from build123d import *

# Parameters (mm, degrees)
SKETCH1_W           = 17.78
SKETCH1_H           = 39.02
BOSS_EXTRUDE1_DEPTH = 2
SKETCH2_R           = 1
CUT_EXTRUDE5_DEPTH  = 10
FILLET4_R           = 7


with BuildPart() as part:
    # Sketch1 → Boss-Extrude1 (new body)
    with BuildSketch(Plane.XY):
        with Locations((8.89, 19.51)):
            Rectangle(SKETCH1_W, SKETCH1_H)
    extrude(amount=BOSS_EXTRUDE1_DEPTH)

    # Sketch2 → Cut-Extrude5 (cut)
    with BuildSketch(Plane.XY.offset(2)):
        with Locations((5.081291963, 2)):
            Circle(SKETCH2_R)
        with Locations((7.621291963, 2)):
            Circle(SKETCH2_R)
        with Locations((10.161291963, 2)):
            Circle(SKETCH2_R)
        with Locations((12.701291963, 2)):
            Circle(SKETCH2_R)
    extrude(amount=-CUT_EXTRUDE5_DEPTH, mode=Mode.SUBTRACT)

    # Fillet4
    fillet4_edges = [part.edges().sort_by_distance(p)[0] for p in [
        (17.78, 0, 1),
        (0, 0, 1),
    ]]
    fillet(fillet4_edges, radius=FILLET4_R)


solid = part.part
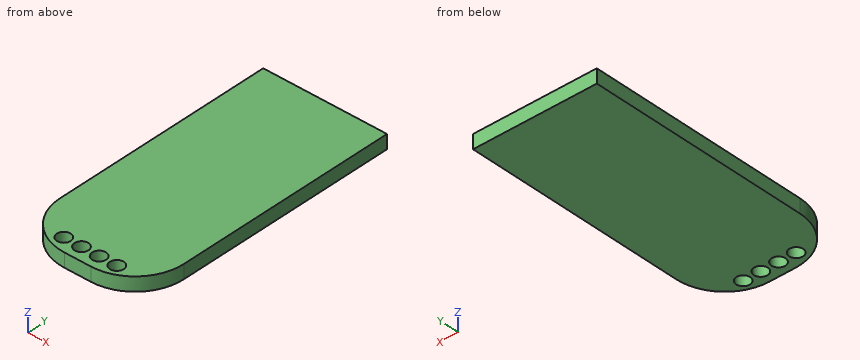
The model under review builds one solid part; all positions refer to its coordinate system, in mm. Round coordinates to 2 decimals unless told otherwise and drop trailing zeros. Loops run counter-clockwise (first coordinate to the right, second up) from the corner with the lowest first, then second, coordinate; pieces in that order, holes last. Notation, with made-up numbers: M -19.5,83 L 2.5,83 A4 ccw 2.5,88 Z; hole C 32,36.25 d11. An arc over 180 degrees is marked long. Answer as CSV lines item,"result".
1. We need section A-A (z = 1.65). Give the boundary of the cut face in (x, y), plus the area to 3 significant figures.
Outcome:
outline,"M 0,7 A7 ccw 7,0 L 10.78,0 A7 ccw 17.78,7 L 17.78,39.02 L 0,39.02 Z; hole C 5.08,2 d2; hole C 7.62,2 d2; hole C 10.16,2 d2; hole C 12.7,2 d2"
area,"660 mm2"
2. We need section C-C (x = 2.75). Give the boundary of the cut face in (y, z).
Outcome:
outline,"M 1.44,0 L 39.02,0 L 39.02,2 L 1.44,2 Z"
3. To check wall thickness, follow L1, parallel to Y at x = 7.75, z = 1.4; L2, parallel to Y at x = 13.5, z = 1; L3, parallel to Y at x = 2.75, z = 1.75. State the ranges of each line that lie inside material, in increasing order. Write a range as [from, to].
Outcome:
L1,"y = [0, 1.01], [2.99, 39.02]"
L2,"y = [0.55, 1.4], [2.6, 39.02]"
L3,"y = [1.44, 39.02]"
4. We need section B-B (y = 2). Give the boundary of the cut face in (x, z).
Outcome:
outline,"M 2.1,0 L 4.08,0 L 4.08,2 L 2.1,2 Z; M 6.08,0 L 6.62,0 L 6.62,2 L 6.08,2 Z; M 8.62,0 L 9.16,0 L 9.16,2 L 8.62,2 Z; M 11.16,0 L 11.7,0 L 11.7,2 L 11.16,2 Z; M 13.7,0 L 15.68,0 L 15.68,2 L 13.7,2 Z"
5. Insertion check: pin 1 Ø1.6 at (x, y) = (12.7, 2) entering from +Z. The pin has a flat end and moves straight along its axis. Give the tip position at first contact, or say it passes through.
Outcome:
pin 1,"passes through"
